```python
from build123d import *

# Parameters (mm, degrees)
BOSS_EXTRUDE1_DEPTH = 2
BOSS_EXTRUDE2_DEPTH = 2
SKETCH3_R           = 3
CUT_EXTRUDE1_DEPTH  = 2
SKETCH4_R           = 1.7
BOSS_EXTRUDE3_DEPTH = 5
CUT_EXTRUDE2_DEPTH  = 1


with BuildPart() as part:
    # Sketch2 → Boss-Extrude1 (new body)
    with BuildSketch(Plane(origin=(0, 0, 0), x_dir=(0, 0, -1), z_dir=(1, 0, 0))):
        Polygon((-8.109308511, -7.091340238), (-8.109308511, 4.696600231), (-4.079902129, 9.498659762), (3.11566899, 9.498659762), (7.090691489, 4.761412419), (7.090691489, -7.091340238), align=None)
    extrude(amount=-BOSS_EXTRUDE1_DEPTH)

    # Sketch1 → Boss-Extrude2 (add)
    with BuildSketch(Plane(origin=(0, 0, 0), x_dir=(0, 0, -1), z_dir=(1, 0, 0))):
        Polygon((-6.109308511, 3.968659762), (-3.147286813, 7.498659762), (-1.232116569, 7.498659762), (-1.232116569, 9.498659762), (-4.079902129, 9.498659762), (-8.109308511, 4.696600231), (-8.109308511, -7.091340238), (-3.982116569, -7.091340238), (-3.982116569, -5.091340238), (-6.109308511, -5.091340238), align=None)
        Polygon((5.090691489, 4.03347195), (5.090691489, -5.091340238), (3.017883431, -5.091340238), (3.017883431, -7.091340238), (7.090691489, -7.091340238), (7.090691489, 4.761412419), (3.11566899, 9.498659762), (0.267883431, 9.498659762), (0.267883431, 7.498659762), (2.183053674, 7.498659762), align=None)
    extrude(amount=BOSS_EXTRUDE2_DEPTH)

    # Sketch3 → Cut-Extrude1 (cut)
    with BuildSketch(Plane(origin=(0, 0, 0), x_dir=(0, 0, -1), z_dir=(1, 0, 0))):
        with Locations((-0.482116569, 1.908659762)):
            Circle(SKETCH3_R)
    extrude(amount=-CUT_EXTRUDE1_DEPTH, mode=Mode.SUBTRACT)

    # Sketch4 → Boss-Extrude3 (add)
    with BuildSketch(Plane(origin=(2, 0, 0), x_dir=(0, 0, -1), z_dir=(1, 0, 0))):
        Polygon((-15.482116569, 1.908659762), (-8.109308511, 1.908659762), (-8.109308511, 4.696600231), (-4.079902129, 9.498659762), (-10.482116569, 9.498659762), (-10.482116569, 17.908659762), (-15.482116569, 17.908659762), align=None)
        with Locations((-12.982116569, 4.408659762)):
            Circle(SKETCH4_R, mode=Mode.SUBTRACT)
        with Locations((-12.982116569, 15.408659762)):
            Circle(SKETCH4_R, mode=Mode.SUBTRACT)
    extrude(amount=-BOSS_EXTRUDE3_DEPTH)

    # Sketch5 → Cut-Extrude2 (cut)
    with BuildSketch(Plane.ZY.offset(3)):
        Polygon((10.482116569, 9.498659762), (10.482116569, 1.908659762), (8.109308511, 1.908659762), (8.109308511, 4.696600231), (4.079902129, 9.498659762), align=None)
    extrude(amount=-CUT_EXTRUDE2_DEPTH, mode=Mode.SUBTRACT)


solid = part.part
```
Here's how the part is built. I have some questions about the finished solid (model axes, mm). A direction names the side the tool comes from. Coordinates: 2 decimals unless noted, no trailing zeros. Loops run counter-clockwise (first coordinate to the right, second up) from the corner with the lowest first, then second, coordinate; pieces in that order, holes last. Notation, with made-up numbers: M 30.5,52.25 L 53.5,52.25 A32 cw 53.5,80.25 Z; hole C -27,7 d5. An arc over 180 degrees is marked long. One line per item, written item: value.
1. Thinking about a two-plate mould opening in Z: for faces 1 (the flat face through (0, 1.909, 12)), 2 (the flat face through (1, -5.091, 5)), 3 (the flat face through (0, 10, 15.482)), which applies, +Z half, -Z half, draft (parallel to the pull), parting line (faces both ways), or undercut?
Geometry says:
face 1: draft
face 2: undercut
face 3: +Z half
2. Imagine slicing it at C-C (z = 2.25). List the corners of the cut face in (x, y) for me, and give its area (3 significant figures).
Geometry says:
outline: M -2,-7.09 L 0,-7.09 L 0,-0.52 L -2,-0.52 Z; M -2,4.33 L 0,4.33 L 0,7.5 L 2,7.5 L 2,9.5 L -2,9.5 Z
area: 27.5 mm2
3. Imagine slicing it at A-A (x = 0.3). List the corners of the cut face in (y, z) for me, and give its area (3 significant figures).
Geometry says:
outline: M -7.09,-7.09 L 4.76,-7.09 L 9.5,-3.12 L 9.5,-0.27 L 7.5,-0.27 L 7.5,-2.18 L 4.03,-5.09 L -5.09,-5.09 L -5.09,-3.02 L -7.09,-3.02 Z; M -7.09,3.98 L -5.09,3.98 L -5.09,6.11 L 3.97,6.11 L 7.5,3.15 L 7.5,1.23 L 9.5,1.23 L 9.5,10.48 L 17.91,10.48 L 17.91,15.48 L 1.91,15.48 L 1.91,8.11 L -7.09,8.11 Z; hole C 4.41,12.98 d3.4; hole C 15.41,12.98 d3.4
area: 175 mm2
4. Please list where these lines run through material, in increasing order: probe 1 along Y at (x, z) = (-2.2, 13.5); probe 2 along Z at (x, y) = (0.3, 0.75); probe 3 along Z at (x, y) = (0.7, 15.5).
Geometry says:
probe 1: y = 1.91 to 2.79, 6.03 to 13.79, 17.03 to 17.91
probe 2: z = -7.09 to -5.09, 6.11 to 8.11
probe 3: z = 10.48 to 11.28, 14.68 to 15.48
5. On a 3-axis mill with a long thin cutter (end or side, diameter ignored), from which of +Z, -Z, +X, -X, +Y, -Y can I reach the whole of each face in a straight line? I mean faces 4 (the flat face through (1, 8, 1.232)), 5 (the flat face through (0, -3, 8.109)), 6 (the flat face through (1, -1, 6.109)), 7 (the flat face through (1, 7.499, 2)). Say none if no direction works.
Geometry says:
face 4: +X, +Y, -Y
face 5: +Z, +X, -X, -Y
face 6: +X
face 7: +X, -Y
6. Imagine slicing it at B-B (y = 1.5). List the corners of the cut face in (x, z) for me, and give its area (3 significant figures).
Geometry says:
outline: M -2,-7.09 L 2,-7.09 L 2,-5.09 L 0,-5.09 L 0,-2.49 L -2,-2.49 Z; M -2,3.45 L 0,3.45 L 0,6.11 L 2,6.11 L 2,8.11 L -2,8.11 Z
area: 26.5 mm2
7. Will these pins go through, and if not, where does the flat tip stop? pin 1 Ø1.2 at (x, y) = (0.5, -3.5) entering from +Z; pin 2 Ø2 at (y, z) = (-4, -0.5) entering from +X; pin 3 Ø1 at (x, z) = (0.5, -4) entering from +Y.
Geometry says:
pin 1: stops at z = 8.11
pin 2: stops at x = 0
pin 3: stops at y = 9.04
8. Imagine slicing it at D-D (y = -5.5). List the corners of the cut face in (x, z) for me, and give its area (3 significant figures).
Geometry says:
outline: M -2,-7.09 L 2,-7.09 L 2,-3.02 L 0,-3.02 L 0,3.98 L 2,3.98 L 2,8.11 L -2,8.11 Z
area: 46.8 mm2
